The listing builds one solid part. Answer for the finished solid, in the listing's coordinates (mm). Face numbers are marked on the shaded views. A direction names the side the tool comes from. Coordinates: 2 decimals unless noted, no trailing zeros. Loops run counter-clockwise (first coordinate to the right, second up) from the corner with the lowest first, then second, coordinate; pieces in that order, holes last. Notation, with made-up numbers: M 60.25,27 L 100.25,27 A14 cw 100.25,42 Z; hole C 9.5,18.25 d4. An arc over 180 degrees is marked long. Answer as a JSON object with one key per item and string values. Group by question number.
1. Straight lines are drawn through the part: L1, parallel to X at y = 14.5, z = -24.25; L2, parallel to Y at x = 36.5, z = -21.5; L3, parallel to Z at x = -7, y = 25.5. For each, find the intervals that lie inside material, in ascending order.
2. A cutting plane is placed at B-B on z = -24.5. Give the vertices of the cut face in (x, y), and give its area (3 significant figures).
3. A cutting plane is placed at C-C on y = 30. Give the vertices of the cut face in (x, z) (3 decimals).
4. A cutting plane is placed at A-A on x = -8. Give the vertices of the cut face in (y, z) (3 decimals), and give its area (3 significant figures).
5. Determine the mould class of the marked faces 1, 2 and 3 for opening direction Y: released by +Y, released by -Y, zero draft, split by the parting line, or undercut.
6. Given pin 1 (2.5 mm diameter, centred on x = 39.5, z = -24, fed in from -Y); pin 2 (2.5 mm diameter, centred on x = -39, z = -22, fed in from +Y); pin 3 (2.5 mm diameter, centred on x = 27.5, z = -31.5, fed in from +Y), each flat-ended and moving along its own axis, determine where each tip first touches the part or whether it passes through.
7. For the marked faces 4, 5, 6 and 7, determine the directions among +Z, -Z, +X, -X, +Y, -Y from which every point of the face is accessible in a straight line to the end or side of a thin tool.
8. A cutting plane is placed at D-D on x = -19. Give the vertices of the cut face in (y, z), and give its area (3 significant figures).
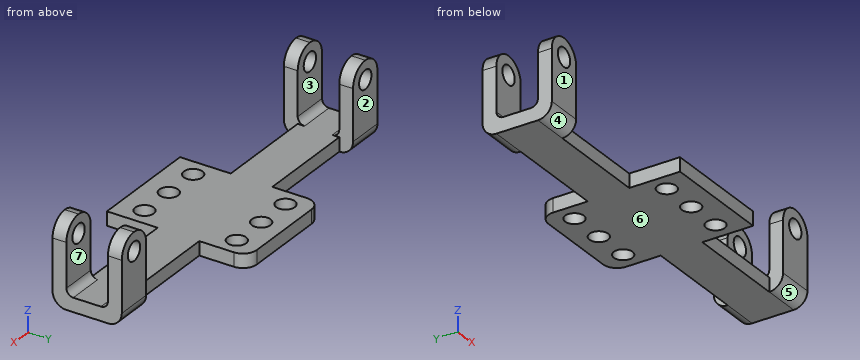
from build123d import *

# Parameters (mm, degrees)
SKETCH1_W                = 40
SKETCH1_H                = 60
BOSS_EXTRUDE1_DEPTH      = 3
BOSS_EXTRUDE3_DEPTH      = 10
BOSS_EXTRUDE3_DEPTH_BACK = 50
SKETCH4_R                = 2.025
CUT_EXTRUDE1_DEPTH       = 76.663729752
SKETCH5_W                = 10
SKETCH5_H                = 3
CUT_EXTRUDE3_DEPTH       = 5
FILLET5_R                = 3
FILLET6_R                = 1.5
SKETCH6_W                = 18
SKETCH6_H                = 30
CUT_EXTRUDE4_DEPTH       = 76.663729752
SKETCH7_W                = 30
SKETCH7_H                = 9
BOSS_EXTRUDE4_DEPTH      = 3
SKETCH8_W                = 8
SKETCH8_H                = 4.5
CUT_EXTRUDE5_DEPTH       = 62.26173357
BOSS_EXTRUDE5_DEPTH      = 15
BOSS_EXTRUDE5_DEPTH_BACK = 3
SKETCH9_W                = 8
SKETCH9_H                = 3
FILLET7_R                = 3
FILLET8_R                = 1.5
SKETCH10_R               = 2.025
CUT_EXTRUDE6_DEPTH       = 16
FILLET9_R                = 4
FILLET10_R               = 3
CUT_EXTRUDE7_DEPTH       = 82.172655494
CUT_EXTRUDE7_DEPTH_BACK  = 10


with BuildPart() as part:
    # Sketch1 → Boss-Extrude1 (new body)
    with BuildSketch(Plane(origin=(0, 0, 0), x_dir=(1, 0, 0), z_dir=(0, 1, 0))):
        Rectangle(SKETCH1_W, SKETCH1_H)
    extrude(amount=BOSS_EXTRUDE1_DEPTH)

    # Sketch3 → Boss-Extrude3 (add, two sides: drawn at the far end of the back side and taken through both)
    with BuildSketch(Plane.ZY.offset(20).offset(-BOSS_EXTRUDE3_DEPTH_BACK)):
        Polygon((-30, 3), (-30, 35), (-33, 35), (-33, 0), (-30, 0), align=None)
    extrude(amount=BOSS_EXTRUDE3_DEPTH + BOSS_EXTRUDE3_DEPTH_BACK)

    # Sketch4 → Cut-Extrude1 (cut, through all)
    with BuildSketch(Plane.XY.offset(-30)):
        with Locations((0, 30)):
            Circle(SKETCH4_R)
        with Locations((8, 30)):
            Circle(SKETCH4_R)
        with Locations((16, 30)):
            Circle(SKETCH4_R)
        with Locations((-8, 30)):
            Circle(SKETCH4_R)
        with Locations((-16, 30)):
            Circle(SKETCH4_R)
        with Locations((-16, 10)):
            Circle(SKETCH4_R)
        with Locations((-8, 10)):
            Circle(SKETCH4_R)
        with Locations((0, 10)):
            Circle(SKETCH4_R)
        with Locations((8, 10)):
            Circle(SKETCH4_R)
        with Locations((16, 10)):
            Circle(SKETCH4_R)
    extrude(amount=-CUT_EXTRUDE1_DEPTH, mode=Mode.SUBTRACT)

    # Sketch5 → Cut-Extrude3 (cut)
    with BuildSketch(Plane.XZ):
        with Locations((-25, -31.5)):
            Rectangle(SKETCH5_W, SKETCH5_H)
        with Locations((25, -31.5)):
            Rectangle(SKETCH5_W, SKETCH5_H)
    extrude(amount=-CUT_EXTRUDE3_DEPTH, mode=Mode.SUBTRACT)

    # Fillet5
    fillet5_edges = [part.edges().sort_by_distance(p)[0] for p in [
        (0, 0, -33),
    ]]
    fillet(fillet5_edges, radius=FILLET5_R)

    # Fillet6
    fillet6_edges = [part.edges().sort_by_distance(p)[0] for p in [
        (0, 3, -30),
    ]]
    fillet(fillet6_edges, radius=FILLET6_R)

    # Sketch6 → Cut-Extrude4 (cut, through all)
    with BuildSketch(Plane.XY.offset(-30)):
        with Locations((-21, 20)):
            Rectangle(SKETCH6_W, SKETCH6_H)
        with Locations((21, 20)):
            Rectangle(SKETCH6_W, SKETCH6_H)
    extrude(amount=-CUT_EXTRUDE4_DEPTH, mode=Mode.SUBTRACT)

    # Sketch7 → Boss-Extrude4 (add)
    with BuildSketch(Plane.XY.offset(-30)):
        with Locations((-27, 20)):
            Rectangle(SKETCH7_W, SKETCH7_H)
        with Locations((27, 20)):
            Rectangle(SKETCH7_W, SKETCH7_H)
    extrude(amount=-BOSS_EXTRUDE4_DEPTH)

    # Sketch8 → Cut-Extrude5 (cut, through all)
    with BuildSketch(Plane(origin=(0, 5, 0), x_dir=(1, 0, 0), z_dir=(0, 1, 0))):
        with Locations((-16, 30.75)):
            Rectangle(SKETCH8_W, SKETCH8_H)
        with Locations((16, 30.75)):
            Rectangle(SKETCH8_W, SKETCH8_H)
    extrude(amount=-CUT_EXTRUDE5_DEPTH, mode=Mode.SUBTRACT)

    # Sketch9 → Boss-Extrude5 (add, two sides: drawn at the far end of the back side and taken through both)
    with BuildSketch(Plane.XY.offset(-30).offset(-BOSS_EXTRUDE5_DEPTH_BACK)):
        with Locations((-38, 26)):
            Rectangle(SKETCH9_W, SKETCH9_H)
        with Locations((-38, 14)):
            Rectangle(SKETCH9_W, SKETCH9_H)
        with Locations((38, 14)):
            Rectangle(SKETCH9_W, SKETCH9_H)
        with Locations((38, 26)):
            Rectangle(SKETCH9_W, SKETCH9_H)
    extrude(amount=BOSS_EXTRUDE5_DEPTH + BOSS_EXTRUDE5_DEPTH_BACK)

    # Fillet7
    fillet7_edges = [part.edges().sort_by_distance(p)[0] for p in [
        (38, 12.5, -33),
        (-38, 12.5, -33),
        (38, 27.5, -33),
        (-38, 27.5, -33),
    ]]
    fillet(fillet7_edges, radius=FILLET7_R)

    # Fillet8
    fillet8_edges = [part.edges().sort_by_distance(p)[0] for p in [
        (-38, 15.5, -30),
        (38, 24.5, -30),
        (-38, 24.5, -30),
        (38, 15.5, -30),
    ]]
    fillet(fillet8_edges, radius=FILLET8_R)

    # Sketch10 → Cut-Extrude6 (cut)
    with BuildSketch(Plane(origin=(0, 27.5, 0), x_dir=(1, 0, 0), z_dir=(0, 1, 0))):
        with Locations(Location((-38, 19, 0), (0, 0, 270))):
            Circle(SKETCH10_R)
        with Locations(Location((38, 19, 0), (0, 0, 180))):
            Circle(SKETCH10_R)
    extrude(amount=-CUT_EXTRUDE6_DEPTH, mode=Mode.SUBTRACT)

    # Fillet9
    fillet9_edges = [part.edges().sort_by_distance(p)[0] for p in [
        (42, 14, -15),
        (42, 26, -15),
        (-34, 14, -15),
        (-34, 26, -15),
        (34, 14, -15),
        (34, 26, -15),
        (-42, 14, -15),
        (-42, 26, -15),
    ]]
    fillet(fillet9_edges, radius=FILLET9_R - 0.0001)  # a hair under: the kernel refuses the full size

    # Fillet10
    fillet10_edges = [part.edges().sort_by_distance(p)[0] for p in [
        (-12, 35, -31.5),
        (12, 35, -31.5),
        (-20, 1.5, -28.5),
        (20, 1.5, -28.5),
        (20, 1.5, 30),
        (-20, 1.5, 30),
    ]]
    fillet(fillet10_edges, radius=FILLET10_R)

    # Sketch11 → Cut-Extrude7 (cut, two sides: drawn at the far end of the back side and taken through both)
    with BuildSketch(Plane.XY.offset(-30).offset(-CUT_EXTRUDE7_DEPTH_BACK)):
        Polygon((-12, 4.5), (-24.843413812, 4.5), (-24.843413812, -2.532189306), (23.385466992, -2.532189306), (23.385466992, 4.5), align=None)
    extrude(amount=CUT_EXTRUDE7_DEPTH + CUT_EXTRUDE7_DEPTH_BACK, mode=Mode.SUBTRACT)


solid = part.part
From the geometry:
{
 "1": {"L1": "x = -42 to -34, 34 to 42", "L2": "y = 12.5 to 15.5, 24.5 to 27.5", "L3": "z = -33 to -30"},
 "2": {"outline": "M -42,12.5 L -34,12.5 L -34,15.5 L -42,15.5 Z; M -42,24.5 L -34,24.5 L -34,27.5 L -42,27.5 Z; M 34,12.5 L 42,12.5 L 42,15.5 L 34,15.5 Z; M 34,24.5 L 42,24.5 L 42,27.5 L 34,27.5 Z", "area": "96.0 mm²"},
 "3": {"outline": "M -12,-33 L -10.025,-33 L -10.025,-30 L -12,-30 Z; M -5.975,-33 L -2.025,-33 L -2.025,-30 L -5.975,-30 Z; M 2.025,-33 L 5.975,-33 L 5.975,-30 L 2.025,-30 Z; M 10.025,-33 L 12,-33 L 12,-30 L 10.025,-30 Z"},
 "4": {"outline": "M 4.5,-33 L 7.975,-33 L 7.975,-30 L 4.5,-30 Z; M 12.025,-33 L 27.975,-33 L 27.975,-30 L 12.025,-30 Z; M 32.025,-33 L 35,-33 L 35,-30 L 32.025,-30 Z", "area": "67.2 mm²"},
 "5": {"face 1": "released by -Y", "face 2": "released by +Y", "face 3": "undercut"},
 "6": {"pin 1": "stops at y = 12.5", "pin 2": "stops at y = 27.5", "pin 3": "stops at y = 24.5"},
 "7": {"face 4": "-Z, -X, -Y", "face 5": "-Z, +X, -Y", "face 6": "-Z, +X, -X, +Y, -Y", "face 7": "+Z, +X, -X"},
 "8": {"outline": "M 15.5,-33 L 24.5,-33 L 24.5,-30 L 15.5,-30 Z", "area": "27.0 mm²"}
}
